CAD build for the part. Positions are in the model's coordinates, mm. Coordinates: 2 decimals unless noted, no trailing zeros. Write each loop counter-clockwise with the first axis right and the second up, starting at its lowest first coordinate (ties: lowest second). Pieces come first, ordered by that corner, then holes. Notation, with made-up numbers: (79, -19.75) -> (131, -19.75) arc R37 ccw to (131, 19.25) -> close; hole circle Ø6 at (-37.5, 70). An arc over 180 degrees is marked (long way). Answer as CSV lines item,"result".
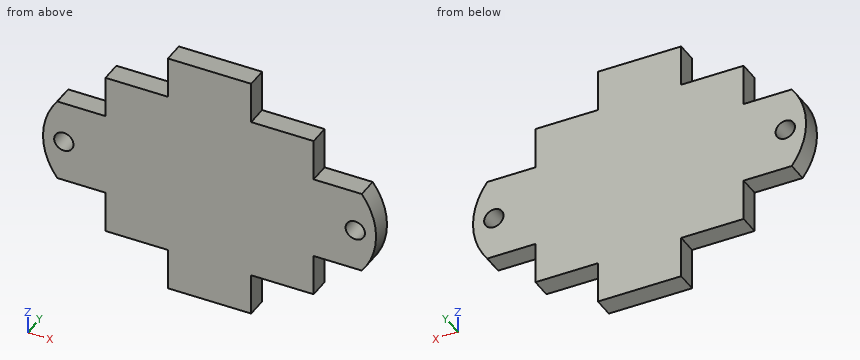
```python
from build123d import *

# Parameters (mm, degrees)
BOSS_EXTRUDE1_DEPTH       = 3.175
F_4_CLEARANCE_HOLE1_D     = 2.9464
F_4_CLEARANCE_HOLE1_DEPTH = 6.35
F_4_CLEARANCE_HOLE1_TIP   = 0.885187864


with BuildPart() as part:
    # Sketch1 → Boss-Extrude1 (new body)
    with BuildSketch(Plane(origin=(0, 0, 0), x_dir=(1, 0, 0), z_dir=(0, 1, 0))):
        with BuildLine():
            Line((-15.875, 12.7), (-6.35, 12.7))
            Line((-6.35, 12.7), (-6.35, 19.05))
            Line((-6.35, 19.05), (6.35, 19.05))
            Line((6.35, 19.05), (6.35, 12.7))
            Line((6.35, 12.7), (15.875, 12.7))
            Line((15.875, 12.7), (15.875, 6.35))
            Line((15.875, 6.35), (19.05, 6.35))
            Line((19.05, 6.35), (23.21476717, 6.35))
            ThreePointArc((23.21476717, 6.35), (25.4, 0), (23.21476717, -6.35))
            Line((23.21476717, -6.35), (19.05, -6.35))
            Line((19.05, -6.35), (15.875, -6.35))
            Line((15.875, -6.35), (15.875, -12.7))
            Line((15.875, -12.7), (6.35, -12.7))
            Line((6.35, -12.7), (6.35, -19.05))
            Line((6.35, -19.05), (-6.35, -19.05))
            Line((-6.35, -19.05), (-6.35, -12.7))
            Line((-6.35, -12.7), (-15.875, -12.7))
            Line((-15.875, -12.7), (-15.875, -6.35))
            Line((-15.875, -6.35), (-19.05, -6.35))
            Line((-19.05, -6.35), (-23.21476717, -6.35))
            ThreePointArc((-23.21476717, -6.35), (-25.4, 0), (-23.21476717, 6.35))
            Line((-23.21476717, 6.35), (-19.05, 6.35))
            Line((-19.05, 6.35), (-15.875, 6.35))
            Line((-15.875, 6.35), (-15.875, 12.7))
        make_face()
    extrude(amount=BOSS_EXTRUDE1_DEPTH)

    # #4 Clearance Hole1
    with Locations(Plane(origin=(0, 3.175, 0), x_dir=(-1, 0, 0), z_dir=(0, 1, 0))):
        with Locations((-22.225, 0), (22.225, 0)):
            Hole(F_4_CLEARANCE_HOLE1_D / 2, depth=F_4_CLEARANCE_HOLE1_DEPTH)
            with Locations((0, 0, -(F_4_CLEARANCE_HOLE1_DEPTH + F_4_CLEARANCE_HOLE1_TIP / 2))):  # 118° drill point
                Cone(0, F_4_CLEARANCE_HOLE1_D / 2, F_4_CLEARANCE_HOLE1_TIP, mode=Mode.SUBTRACT)


solid = part.part
```
Item 1: Saw through at B-B on y = 2.1. State how many separate pieces and enclosed holes the cut face has, and give its area (3 significant figures).
Answer below:
separate pieces,"1"
enclosed holes,"2"
area,"1,180 mm2"
Item 2: Flat gauge pins, fed straight in: pin 1 (1.5 mm diameter, centred on y = 1, z = 11.5, fed in from -X) (3 decimals); pin 2 (1.6 mm diameter, centred on x = 9.5, y = 1, fed in from -Z); pin 3 (1.6 mm diameter, centred on y = 1, z = -15.5, fed in from -X). Where does each tip first touch, or does it go through?
Answer below:
pin 1,"stops at x = -15.875"
pin 2,"stops at z = -12.7"
pin 3,"stops at x = -6.35"
Item 3: Saw through at D-D on z = -14.5. Give the cut face in (x, y) (3 decimals), and give its area (3 significant figures).
Answer below:
outline,"(-6.35, 0) -> (6.35, 0) -> (6.35, 3.175) -> (-6.35, 3.175) -> close"
area,"40.3 mm2"
Item 4: Saw through at C-C on x = 18. Give the cut face in (y, z) (3 decimals).
Answer below:
outline,"(0, -6.35) -> (3.175, -6.35) -> (3.175, 6.35) -> (0, 6.35) -> close"
Item 5: Wall check: line 1 (X direction, y = 1.6, z = -10) (3 decimals); line 2 (Z direction, x = 13.5, y = 1.1); line 3 (Z direction, x = 17.5, y = 1.2). Give the ranges that are in metal, low to high. Write a range as from..to.
Answer below:
line 1,"x = -15.875..15.875"
line 2,"z = -12.7..12.7"
line 3,"z = -6.35..6.35"
Item 6: Saw through at A-A on z = 0. Give the cut face in (x, y) (3 decimals), and give its area (3 significant figures).
Answer below:
outline,"(-25.4, 0) -> (-23.698, 0) -> (-23.698, 3.175) -> (-25.4, 3.175) -> close; (-20.752, 0) -> (20.752, 0) -> (20.752, 3.175) -> (-20.752, 3.175) -> close; (23.698, 0) -> (25.4, 0) -> (25.4, 3.175) -> (23.698, 3.175) -> close"
area,"143 mm2"
